Model file for the job. Use its own axes, mm. A direction names the side the tool comes from. Round coordinates to 2 decimals unless told otherwise and drop trailing zeros. Loops run counter-clockwise (first coordinate to the right, second up) from the corner with the lowest first, then second, coordinate; pieces in that order, holes last. Notation, with made-up numbers: (41, 26.5) - (70, 26.5) arc R31 ccw to (70, 54.5) - close; hole circle Ø1 at (-3.75, -15). An arc over 180 degrees is marked (long way). Use one line per item in the form item = value.
Autodesk Inventor part; units mm, degrees
ref_plane "YZ Plane" through (0, 0, 0) normal (1, 0, 0) x (0, 1, 0)
ref_plane "XZ Plane" through (0, 0, 0) normal (0, 1, 0) x (-1, 0, 0)
ref_plane "XY Plane" through (0, 0, 0) normal (0, 0, 1) x (1, 0, 0)
sketch "スケッチ1" plane through (0, 0, 0) normal (1, 0, 0) x (0, 1, 0)
  line L0 (0, 0) -> (100, 0)
  line L1 (100, 0) -> (100, 10)
  line L2 (20, 90) -> (0, 90)
  line L3 (0, 90) -> (0, 0)
  line L4 (100, 10) -> (80, 10)
  line L5 (80, 10) -> (80, 30)
  line L6 (80, 30) -> (20, 30)
  line L7 (20, 30) -> (20, 90)
  dimension "d0" = 100
  dimension "d1" = 10
  dimension "d23" = 20
  dimension "d24" = 20
  dimension "d25" = 80
  dimension "d26" = 90
extrude "押し出し1" add sketch "スケッチ1" along normal mid plane 40
fillet "フィレット1" radius 30 1 edges at (0, 20, 30)
sketch "スケッチ2" plane through (-20, 100, 10) normal (0, 1, 0) x (1, 0, 0)
  line L0 (0, -80) -> (40, -80)
  line L1 (40, -20) -> (0, -20)
  line L2 (5, -20) -> (35, -20)
  line L3 (35, -20) -> (35, -75)
  line L4 (35, -75) -> (5, -75)
  line L5 (5, -75) -> (5, -20)
  line L6 (0, -20) -> (0, -50)
  line L7 (40, -50) -> (40, -80)
  dimension "d27" = 5
  dimension "d28" = 5
  dimension "d29" = 5
extrude "押し出し2" cut sketch "スケッチ2" against normal blind 90
sketch "スケッチ3" plane through (20, 100, 0) normal (0, 0, -1) x (-1, 0, 0)
  line L0 (40, 0) -> (0, 0)
  line L1 (0, -100) -> (0, 0)
  line L2 (40, 0) -> (40, -100)
  point P0 (20, -100)
  point P1 (7, -10)
  point P2 (33, -10)
  dimension "d12" = 10
  dimension "d13" = 10
  dimension "d14" = 7
  dimension "d15" = 7
hole "穴1" at (13, 90, 0) at (-13, 90, 0) direction (0, 0, 1) diameter 5.2 end through all
equation "\"d28\" = d27"
equation "\"d29\" = d27"
properties part number "s_base8"
1. Cut at A-A, the plane y = 90. Give the cut face in (x, z), plus the area to 3 significant figures.
Geometry check:
outline = (-20, 0) - (-15.6, 0) - (-15.6, 10) - (-20, 10) - close; (-10.4, 0) - (10.4, 0) - (10.4, 10) - (-10.4, 10) - close; (15.6, 0) - (20, 0) - (20, 10) - (15.6, 10) - close
area = 296 mm^2
2. Cut at B-B, the plane x = 13. Give the cut face in (y, z), plus the area to 3 significant figures.
Geometry check:
outline = (0, 0) - (87.4, 0) - (87.4, 10) - (80, 10) - (80, 30) - (10, 30) - (10, 85) - (20, 85) - (20, 90) - (0, 90) - close; (92.6, 0) - (100, 0) - (100, 10) - (92.6, 10) - close
area = 3,200 mm^2
3. Wall check: probe 1 along X at (y, z) = (90, 2); probe 2 along Y at (x, z) = (-13, 3); probe 3 along X at (y, z) = (21, 47). Give the ranges that are in metal, low to high.
Geometry check:
probe_1 = -20 to -15.6, -10.4 to 10.4, 15.6 to 20
probe_2 = 0 to 87.4, 92.6 to 100
probe_3 = -20 to -15, 15 to 20
4. Flat gauge pins, fed straight in: pin 1 (20 mm diameter, centred on x = 1, y = 56.5, fed in from +Z); pin 2 (9 mm diameter, centred on x = 1, z = 79, fed in from +Y); pin 3 (22 mm diameter, centred on x = 7.5, z = 18, fed in from +Y); pin 4 (6 mm diameter, centred on x = -10, z = 16.5, fed in from +Y). Where does each tip first touch, or does it go through?
Geometry check:
pin_1 = 30
pin_2 = 10
pin_3 = 100
pin_4 = 80
5. Pull direction Y, two halves, no side cores. Call faces 4 (the cylindrical face through (17.465, 29.021, 38.555)), 5 (the cylindrical face through (-13.1, 87.4, 5.1)), 6 (the cylindrical face through (12.9, 87.4, 5.1)), 7 (the flat face through (0, 90, 10)): +Y half, -Y half, draft (parallel to the pull), parting line (faces both ways), or undercut.
Geometry check:
face_4 = +Y half
face_5 = undercut
face_6 = undercut
face_7 = draft
6. Cut at C-C, the plane y = 12.5. Give the cut face in (x, z), plus the area to 3 significant figures.
Geometry check:
outline = (-20, 0) - (20, 0) - (20, 90) - (-20, 90) - close; hole (-15, 30) - (15, 30) - (15, 85) - (-15, 85) - close
area = 1,950 mm^2
7. Tool access for faces 1 (the flat face through (0, 20, 86)), 2 (the flat face through (0, 0, 46)), 3 (the flat face through (15, 18, 53)): list every direction of +Z, -Z, +X, -X, +Y, -Y with a clear straight run to the whole face (end or side of a thin tool).
Geometry check:
face_1 = +Z, +X, -X, +Y
face_2 = +Z, -Z, +X, -X, -Y
face_3 = +Y
8. Cut at D-D, the plane z = 39. Give the cut face in (x, y), plus the area to 3 significant figures.
Geometry check:
outline = (-20, 0) - (20, 0) - (20, 28.58) - (15, 28.58) - (15, 10) - (-15, 10) - (-15, 28.58) - (-20, 28.58) - close
area = 586 mm^2
